For this review, use the dimensioned drawing (mm, ordinates from the lowest corner) and the shaded views. A direction names the side the tool comes from. Round coordinates to 2 decimals unless told otherwise and drop trailing zeros. Write each loop counter-clockwise with the first axis right and the second up, starting at its lowest first coordinate (ties: lowest second). Pieces come first, ordered by that corner, then holes.
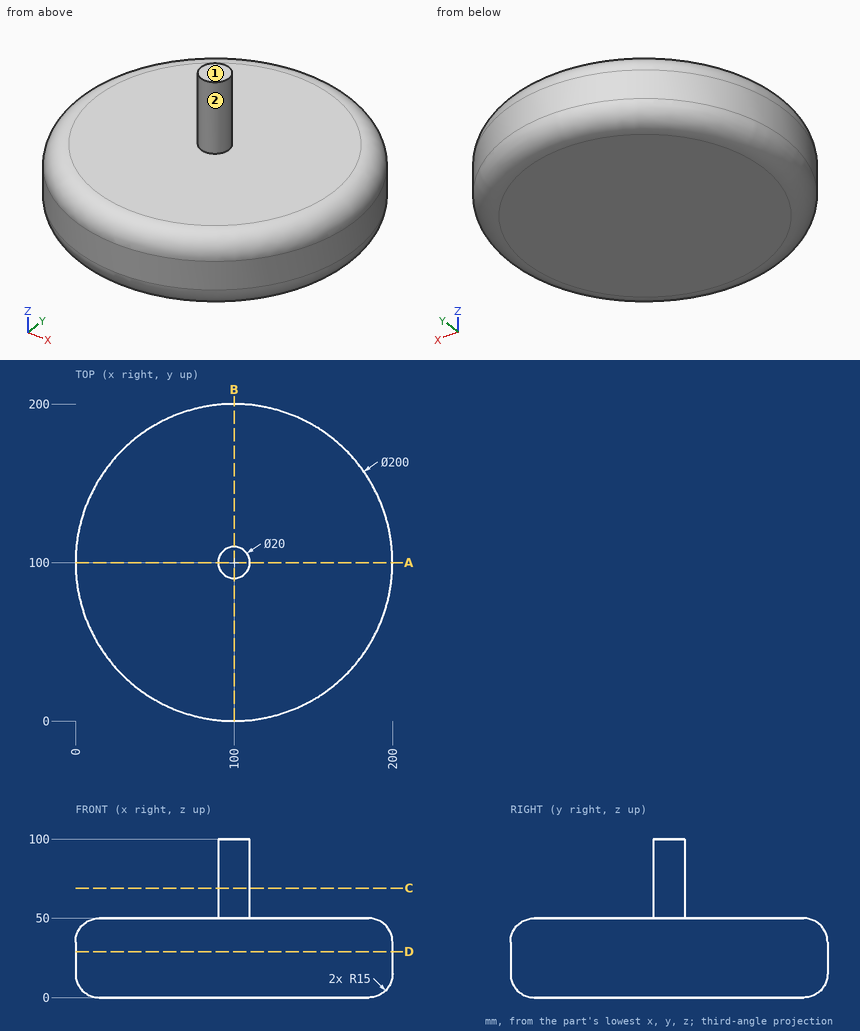
(1) For line 1 along Z through (x, y) = (83.5, 82); line 2 along Y through (x, z) = (174.5, 10); line 3 along X through (y, z) = (133, 28), list the stretches that pass through material, from the lowest coordinate up.
Geometry check:
line 1: z = 0 to 50
line 2: y = 34.59 to 165.41
line 3: x = 5.6 to 194.4
(2) For pin 1 Ø2 at (y, z) = (103.5, 60.5) entering from +X; pin 2 Ø1 at (y, z) = (88, 45) entering from +X; pin 3 Ø1 at (x, z) = (105.5, 46.5) entering from -Y, all flat-tipped, find the tip position at first contact; note any pin that passes through.
Geometry check:
pin 1: stops at x = 109.68
pin 2: stops at x = 195.86
pin 3: stops at y = 4.96
(3) We need section A-A, the plane y = 100. Give the boundary of the cut face in (x, z).
Geometry check:
outline: (0, 15) arc R15 ccw to (15, 0) - (185, 0) arc R15 ccw to (200, 15) - (200, 35) arc R15 ccw to (185, 50) - (110, 50) - (110, 100) - (90, 100) - (90, 50) - (15, 50) arc R15 ccw to (0, 35) - close
(4) For the marked faces 1 and 2, list the 3-axis set-ups (+Z, -Z, +X, -X, +Y, -Y) from which the entire face can be reached by the end or side of a thin tool; tool diameter is ignored.
Geometry check:
face 1: +Z, +X, -X, +Y, -Y
face 2: +Z
(5) We need section D-D, the plane z = 29. Give the boundary of the cut face in (x, y).
Geometry check:
outline: circle Ø200 at (100, 100)
(6) We need section C-C, the plane z = 69. Give the boundary of the cut face in (x, y).
Geometry check:
outline: circle Ø20 at (100, 100)
